Part print with two shaded views. Sizes in mm from the minimum x, y, z corner. Give positions to 0.01 mm unless a question says otherwise; leave off trailing zeros. Write each loop counter-clockwise with the first axis right and the second up, starting at its lowest first coordinate (ties: lowest second). Pieces come first, ordered by that corner, then holes. Notation, with made-up numbers: M -24.5,33.5 L 8.5,33.5 A19 ccw 8.5,66.5 Z; hole C -33,-28.5 d4. An arc over 180 degrees is marked long. Return JSON: item names as keys, results as strings. Group by question number.
Q1. Wall check: probe 1 along Y at (x, z) = (10.5, 16.5); probe 2 along X at (y, z) = (42, 16.5); probe 3 along Z at (x, y) = (29, 17). Give the ranges that are in metal, low to high.
Q2. Flat gauge pins, fed straight in: pin 1 Ø6 at (y, z) = (125, 5) entering from -X; pin 2 Ø3 at (x, y) = (19, 51.5) entering from +Z. Where does each tip first touch, or does it go through?
Q3. Pull direction X, two halves, no side cores. Call the marked faces 1 and 2: +X half, -X half, draft (parallel to the pull), parting line (faces both ways), or undercut.
Q4. Band-saw the part on C-C, the plane x = 10.5. Give the cut face in (y, z) (3 decimals), then the cut area to 3 significant figures.
Q5. Band-saw the part on A-A, the plane y = 108. Give the cut face in (x, z).
Q6. Band-saw the part on B-B, the plane z = 18.75. Give the cut face in (x, y).
Q7. Band-saw the part on D-D, the plane y = 60.5. Give the cut face in (x, z).
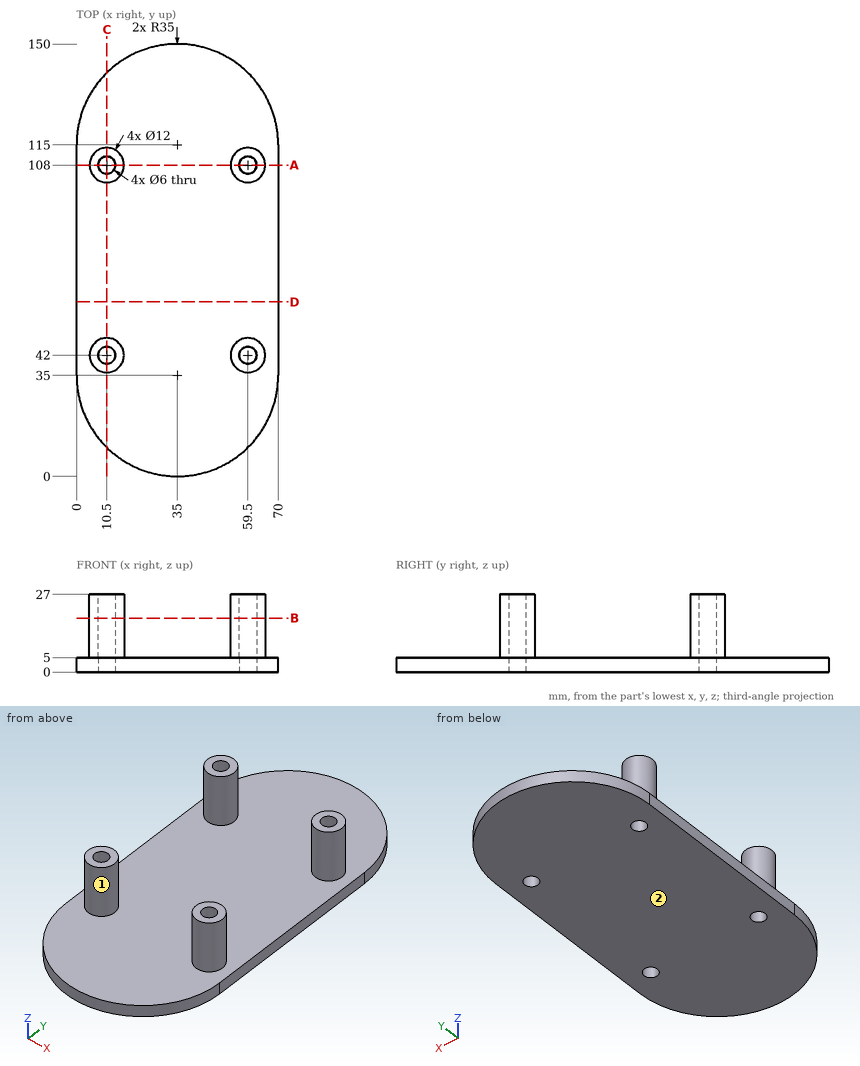
From the geometry:
{
 "1": {"probe 1": "y = 36 to 39, 45 to 48, 102 to 105, 111 to 114", "probe 2": "x = 4.5 to 7.5, 13.5 to 16.5, 53.5 to 56.5, 62.5 to 65.5", "probe 3": "z = 0 to 5"},
 "2": {"pin 1": "stops at x = 0.71", "pin 2": "stops at z = 5"},
 "3": {"face 1": "undercut", "face 2": "draft"},
 "4": {"outline": "M 10.005,0 L 39,0 L 39,27 L 36,27 L 36,5 L 10.005,5 Z; M 45,0 L 105,0 L 105,27 L 102,27 L 102,5 L 48,5 L 48,27 L 45,27 Z; M 111,0 L 139.995,0 L 139.995,5 L 114,5 L 114,27 L 111,27 Z", "area": "854 mm^2"},
 "5": {"outline": "M 0,0 L 7.5,0 L 7.5,27 L 4.5,27 L 4.5,5 L 0,5 Z; M 13.5,0 L 56.5,0 L 56.5,27 L 53.5,27 L 53.5,5 L 16.5,5 L 16.5,27 L 13.5,27 Z; M 62.5,0 L 70,0 L 70,5 L 65.5,5 L 65.5,27 L 62.5,27 Z"},
 "6": {"outline": "C 10.5,42 d12; C 10.5,108 d12; C 59.5,42 d12; C 59.5,108 d12; hole C 10.5,42 d6; hole C 10.5,108 d6; hole C 59.5,42 d6; hole C 59.5,108 d6"},
 "7": {"outline": "M 0,0 L 70,0 L 70,5 L 0,5 Z"}
}
